Geometry check sheet. Reference: the model listing, model coordinates, mm. Coordinates: 2 decimals unless noted, no trailing zeros. Order: outer loops, then holes, each group sorted by start corner. A loop starts at its lowest first (then second) coordinate and runs counter-clockwise, first axis right, second up. Notation, with made-up numbers: M 66.5,4 L 83.5,4 A34 ccw 83.5,34 Z; hole C 11.25,-35.5 d11. An arc over 180 degrees is marked long. One line per item, written item: value. Start each with the question number.
1) Go/stop test with flat-tipped pins: P1, Ø4, axis at x = 19, y = 513.5, coming from the +Z side; P2, Ø1.5, axis at y = 166.5, z = 8.5, coming from the +X side; P3, Ø10, axis at x = -7.5, y = 661, coming from the -Z side. Record where each tip stops, or that it passes through.
2) Sectioned sample at B-B, the plane y = 740. Enter the section's corners in (x, z) (3 decimals), then the cut area to 3 significant figures.
3) Sectioned sample at A-A, the plane x = 0. Enter the section's corners in (y, z) (3 decimals).
4) Thickness scan on L1, parallel to X at y = 576.5, z = 0 (3 decimals); L2, parallel to X at y = 392.5, z = -6; L3, parallel to Z at x = 8.5, y = 445. Record the ranges inside material, lowest first. Write a range as from..to.
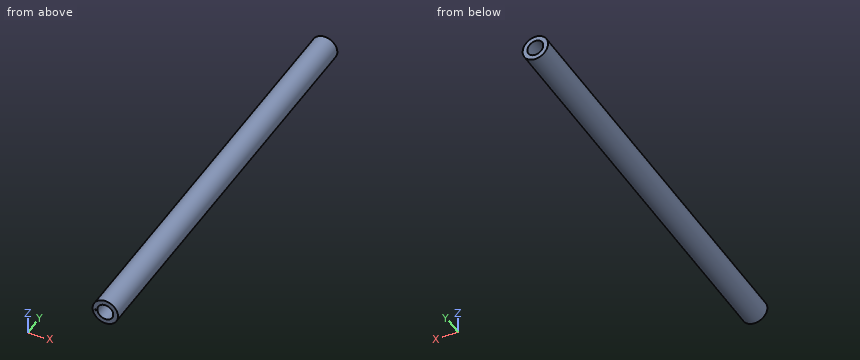
```python
from build123d import *

# Parameters (mm, degrees)
SKETCH1_R           = 25.4
SKETCH1_R_2         = 15.875
BOSS_EXTRUDE1_DEPTH = 838.2
CUT_EXTRUDE3_DEPTH  = 5.08


with BuildPart() as part:
    # Sketch1 → Boss-Extrude1 (new body)
    with BuildSketch(Plane(origin=(0, 0, 0), x_dir=(1, 0, 0), z_dir=(0, 1, 0))):
        with Locations(Location((0, 0, 0), (0, 0, 270))):
            Circle(SKETCH1_R)
        with Locations(Location((0, 0, 0), (0, 0, 270))):
            Circle(SKETCH1_R_2, mode=Mode.SUBTRACT)
    extrude(amount=BOSS_EXTRUDE1_DEPTH)

    # Sketch5 → Cut-Extrude3 (cut)
    with BuildSketch(Plane.XZ):
        with BuildLine():
            Line((-20.9422761, -0.95712788), (-20.322794931, -0.95712788))
            add(Edge.make_bspline(
                [(-20.322794931, -0.95712788), (-20.292470525, -0.957287311), (-20.233694281, -0.957596328), (-20.148223787, -0.962388882), (-20.068169509, -0.96892364), (-19.99350823, -0.979292367), (-19.92427445, -0.991803479), (-19.860259522, -1.006954412), (-19.801667008, -1.025121412), (-19.73171474, -1.054010538), (-19.651958141, -1.096939412), (-19.565599599, -1.160374611), (-19.491754325, -1.237964774), (-19.428085308, -1.325488325), (-19.377465721, -1.421768633), (-19.340845001, -1.524510897), (-19.317660357, -1.632389906), (-19.315275992, -1.706451931), (-19.314070972, -1.743881687)],
                knots=[0, 0, 0, 0, 1.001505555, 1.941167018, 2.826882275, 3.653841531, 4.429895133, 5.150066043, 5.825578002, 6.45369114, 7.647487171, 8.808567382, 9.977351308, 11.170798116, 12.373658725, 13.556498008, 14.765093433, 16, 16, 16, 16], degree=3))
            add(Edge.make_bspline(
                [(-19.314070972, -1.743881687), (-19.315062678, -1.778945076), (-19.317011472, -1.847847944), (-19.335646689, -1.948626172), (-19.36482101, -2.044557634), (-19.405375057, -2.135292227), (-19.458081868, -2.218779862), (-19.5205462, -2.295694024), (-19.595908728, -2.362778198), (-19.652372239, -2.400282116), (-19.681053144, -2.419332408)],
                knots=[0, 0, 0, 0, 1.044552857, 2.05264487, 3.044412934, 4.028983338, 5.005914585, 5.980388656, 6.974128949, 8, 8, 8, 8], degree=3))
            add(Edge.make_bspline(
                [(-19.681053144, -2.419332408), (-19.644984756, -2.433179942), (-19.575976995, -2.459673707), (-19.481011827, -2.506514449), (-19.399192217, -2.557461506), (-19.329889092, -2.613098256), (-19.270618505, -2.673068392), (-19.218863336, -2.738251245), (-19.174702376, -2.809497119), (-19.136862795, -2.886063183), (-19.107336423, -2.967167622), (-19.085223996, -3.052049683), (-19.072553524, -3.140404994), (-19.07075045, -3.200535302), (-19.069840203, -3.230890901)],
                knots=[0, 0, 0, 0, 1.27268992, 2.434971085, 3.483601985, 4.442670788, 5.356604649, 6.2567628, 7.179492994, 8.113709626, 9.066344395, 10.018646069, 10.999752585, 12, 12, 12, 12], degree=3))
            add(Edge.make_bspline(
                [(-19.069840203, -3.230890901), (-19.070726342, -3.261885135), (-19.072469845, -3.322867159), (-19.085333105, -3.412452174), (-19.107112795, -3.498063733), (-19.137113049, -3.580255577), (-19.176267435, -3.658868699), (-19.223917802, -3.73399216), (-19.280733578, -3.80487116), (-19.344290609, -3.872293304), (-19.416192698, -3.932915654), (-19.493767704, -3.986904902), (-19.57799258, -4.031305972), (-19.667484032, -4.068604078), (-19.763245947, -4.097094893), (-19.864848313, -4.117027157), (-19.972203501, -4.13045744), (-20.045872346, -4.131561619), (-20.083652302, -4.13212788)],
                knots=[0, 0, 0, 0, 0.978564426, 1.925352924, 2.850884081, 3.763762016, 4.682927383, 5.618979971, 6.567305752, 7.547517671, 8.540179244, 9.531824382, 10.526200242, 11.540722885, 12.589160233, 13.674978461, 14.80764778, 16, 16, 16, 16], degree=3))
            Line((-20.083652302, -4.13212788), (-20.9422761, -4.13212788))
            Line((-20.9422761, -4.13212788), (-20.9422761, -0.95712788))
        make_face()
        with BuildLine():
            Line((-20.657340203, -1.282768906), (-20.657340203, -2.300397111))
            Line((-20.657340203, -2.300397111), (-20.465898897, -2.300397111))
            add(Edge.make_bspline(
                [(-20.465898897, -2.300397111), (-20.437914633, -2.300034324), (-20.383843331, -2.299333345), (-20.305538853, -2.297325369), (-20.232854015, -2.291702858), (-20.165914281, -2.286081963), (-20.104825064, -2.276942873), (-20.049721704, -2.266064304), (-19.999739405, -2.254559097), (-19.94209996, -2.234992491), (-19.8767195, -2.206074886), (-19.807020898, -2.161196863), (-19.745576058, -2.107744057), (-19.693690038, -2.046066542), (-19.651225347, -1.978152216), (-19.621730762, -1.905084689), (-19.601730726, -1.828684998), (-19.599924123, -1.776235583), (-19.59900687, -1.749605845)],
                knots=[0, 0, 0, 0, 1.156816544, 2.235205308, 3.236616184, 4.169592532, 5.011045266, 5.787822928, 6.49130361, 7.128639758, 8.301311294, 9.436451833, 10.541879658, 11.654887649, 12.756523258, 13.837046038, 14.901820046, 16, 16, 16, 16], degree=3))
            add(Edge.make_bspline(
                [(-19.59900687, -1.749605845), (-19.59948419, -1.731983895), (-19.600420507, -1.697416516), (-19.60808886, -1.647025317), (-19.621122302, -1.59963277), (-19.637862983, -1.554589398), (-19.661257007, -1.513303648), (-19.688801006, -1.474348035), (-19.722080168, -1.439049185), (-19.759960016, -1.406056854), (-19.803510695, -1.376806461), (-19.852706224, -1.351188054), (-19.908212189, -1.330558921), (-19.969093136, -1.312492126), (-20.036286194, -1.299802745), (-20.109015967, -1.289231458), (-20.187878176, -1.283849613), (-20.242438377, -1.283137177), (-20.270641485, -1.282768906)],
                knots=[0, 0, 0, 0, 0.91205012, 1.789085906, 2.630437955, 3.453916878, 4.269457761, 5.079663411, 5.91843418, 6.774407191, 7.675494373, 8.627863946, 9.638891023, 10.736472738, 11.911756761, 13.175263542, 14.539845004, 16, 16, 16, 16], degree=3))
            Line((-20.270641485, -1.282768906), (-20.657340203, -1.282768906))
        make_face(mode=Mode.SUBTRACT)
        with BuildLine():
            Line((-20.657340203, -2.626038137), (-20.657340203, -3.806486855))
            Line((-20.657340203, -3.806486855), (-20.251560956, -3.806486855))
            add(Edge.make_bspline(
                [(-20.251560956, -3.806486855), (-20.222515216, -3.806138741), (-20.166533382, -3.805467798), (-20.085705837, -3.803277452), (-20.010791164, -3.798295173), (-19.942131213, -3.790452152), (-19.878984588, -3.781944559), (-19.822108814, -3.770504326), (-19.771042846, -3.757397055), (-19.711829724, -3.73713677), (-19.645151542, -3.705662114), (-19.573295979, -3.658205637), (-19.509409338, -3.601669494), (-19.455157425, -3.53623645), (-19.410695642, -3.465088032), (-19.378351051, -3.389663322), (-19.358402202, -3.311208593), (-19.355987234, -3.257717361), (-19.3547761, -3.230890901)],
                knots=[0, 0, 0, 0, 1.160039823, 2.235823828, 3.228722157, 4.157150951, 4.99529583, 5.772374946, 6.472645482, 7.099169577, 8.269452708, 9.405989375, 10.527446681, 11.663510218, 12.788923519, 13.866172445, 14.929861265, 16, 16, 16, 16], degree=3))
            add(Edge.make_bspline(
                [(-19.3547761, -3.230890901), (-19.355026567, -3.2141148), (-19.355523459, -3.180833196), (-19.363017016, -3.131923846), (-19.373915313, -3.084547518), (-19.388004542, -3.038575568), (-19.40852363, -2.994839148), (-19.432478139, -2.952473254), (-19.460564553, -2.911421884), (-19.504328903, -2.859522197), (-19.567984918, -2.799726049), (-19.658433207, -2.741181315), (-19.761278077, -2.693966519), (-19.83587016, -2.673919136), (-19.874402503, -2.663563177)],
                knots=[0, 0, 0, 0, 0.723448775, 1.435228256, 2.130040452, 2.821711965, 3.505591119, 4.210454504, 4.921174351, 5.648778258, 7.137944449, 8.670945889, 10.280296675, 12, 12, 12, 12], degree=3))
            add(Edge.make_bspline(
                [(-19.874402503, -2.663563177), (-19.889850325, -2.660428922), (-19.923344391, -2.653633211), (-19.977961268, -2.646459795), (-20.04031452, -2.640068919), (-20.11054813, -2.635341655), (-20.188750958, -2.63045529), (-20.27509002, -2.628554988), (-20.369212726, -2.626287802), (-20.434520093, -2.626123488), (-20.468442967, -2.626038137)],
                knots=[0, 0, 0, 0, 0.634451884, 1.375622551, 2.216452059, 3.157844607, 4.20941857, 5.370758133, 6.634282058, 8, 8, 8, 8], degree=3))
            Line((-20.468442967, -2.626038137), (-20.657340203, -2.626038137))
        make_face(mode=Mode.SUBTRACT)
    extrude(amount=-CUT_EXTRUDE3_DEPTH, mode=Mode.SUBTRACT)


solid = part.part
```
Final values:
1. P1: stops at z = 18.87
1. P2: stops at x = 24.19
1. P3: stops at z = -25.28
2. outline: C 0,0 d50.8; hole C 0,0 d31.75
2. area: 1,240 mm^2
3. outline: M 0,-25.4 L 838.2,-25.4 L 838.2,-15.875 L 0,-15.875 Z; M 0,15.875 L 838.2,15.875 L 838.2,25.4 L 0,25.4 Z
4. L1: x = -25.4..-15.875, 15.875..25.4
4. L2: x = -24.68..-14.7, 14.7..24.68
4. L3: z = -23.94..-13.41, 13.41..23.94
